CAD build for the part. Positions are in the model's coordinates, mm. Face numbers are marked on the shaded views. A direction names the side the tool comes from. Give positions to 0.01 mm unless a question says otherwise; leave off trailing zeros. Order: outer loops, then holes, each group sorted by start corner. A loop starts at its lowest first (then second) coordinate and runs counter-clockwise, first axis right, second up.
Item 1: Band-saw the part on B-B on y = 12. Give the cut face in (x, z), plus the area to 3 significant figures.
Item 2: Wall check: L1, parallel to X at y = -5.5, z = 15; L2, parallel to Y at x = 93.5, z = 23.5; L3, parallel to Y at x = -69, z = 2.25. Give the ranges that are in metal, low to high.
Item 3: Band-saw the part on A-A on z = 15. Give the cut face in (x, y).
Item 4: Which spindle directions (+Z, -Z, +X, -X, +Y, -Y) get a long thin tool onto all of the face, cutting with end or side? Do the marked faces 5, 6 and 7. Say none if no direction does.
Item 5: Band-saw the part on D-D on x = -52. Give the cut face in (y, z), plus the area to 3 significant figures.
Item 6: Flat gauge pins, fed straight in: P1, Ø5, axis at y = 53.5, z = 6.5, coming from the -X side; P2, Ø11, axis at y = 19, z = 7, coming from the +X side; P3, Ø1.5, axis at y = 42, z = 24.5, coming from the -X side; P4, Ø10, axis at x = 42, y = 9.5, coming from the +Z side. Where does each tip first touch, or does it go through?
Item 7: Band-saw the part on C-C on z = 5. Give the cut face in (x, y), plus the area to 3 significant figures.
Item 8: Two-plate mould, pull along Y, no slides. Class the marked faces 1, 2, 3 and 4: released by +Y, released by -Y, zero draft, split by the parting line, or undercut.
```python
from build123d import *

# Parameters (mm, degrees)
BOSS_EXTRUDE1_DEPTH = 30
SKETCH2_R           = 5
CUT_EXTRUDE1_DEPTH  = 90


with BuildPart() as part:
    # Sketch1 → Boss-Extrude1 (new body)
    with BuildSketch(Plane.XY):
        Polygon((-77.503184713, 15), (-77.503184713, -15), (102.496815287, -15), (102.496815287, 0), (72.496815287, 0), (72.496815287, 70.165605096), (102.496815287, 70.165605096), (102.496815287, 85.165605096), (52.496815287, 85.165605096), (-47.503184713, 15), align=None)
        with BuildLine():
            Line((52.496815287, 50.932984608), (52.496815287, 10))
            ThreePointArc((52.496815287, 10), (49.567883098, 2.928932188), (42.496815287, 0))
            Line((42.496815287, 0), (-15.840862486, 0))
            ThreePointArc((-15.840862486, 0), (-25.376570483, 6.988310608), (-21.58458061, 18.185945401))
            Line((-21.58458061, 18.185945401), (36.753097163, 59.11893001))
            ThreePointArc((36.753097163, 59.11893001), (47.109993083, 59.805334388), (52.496815287, 50.932984608))
        make_face(mode=Mode.SUBTRACT)
    extrude(amount=BOSS_EXTRUDE1_DEPTH)

    # Sketch2 → Cut-Extrude1 (cut, symmetric)
    with BuildSketch(Plane(origin=(0, 15, 0), x_dir=(1, 0, 0), z_dir=(0, 1, 0))):
        with Locations(Location((-62.503184713, -15, 0), (0, 0, 270))):
            Circle(SKETCH2_R)
        with Locations(Location((72.496815287, -15, 0), (0, 0, 270))):
            Circle(SKETCH2_R)
    extrude(amount=CUT_EXTRUDE1_DEPTH, both=True, mode=Mode.SUBTRACT)


solid = part.part
```
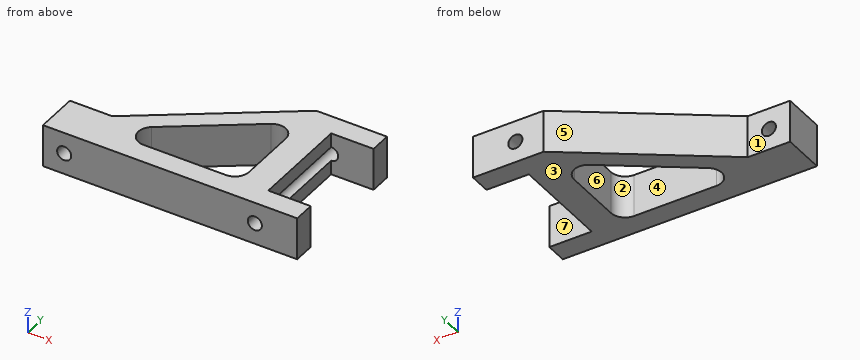
The answers:
1. outline: (-77.5, 0) - (-25.64, 0) - (-25.64, 30) - (-77.5, 30) - close; (52.5, 0) - (72.5, 0) - (72.5, 10) arc R5 cw to (72.5, 20) - (72.5, 30) - (52.5, 30) - close; hole circle Ø10 at (-62.5, 15)
1. area: 2,040 mm2
2. L1: x = -77.5 to -67.5, -57.5 to 67.5, 77.5 to 102.5
2. L2: y = -15 to 0, 70.17 to 85.17
2. L3: y = -15 to 15
3. outline: (-77.5, -15) - (-67.5, -15) - (-67.5, 15) - (-77.5, 15) - close; (-57.5, -15) - (67.5, -15) - (67.5, 85.17) - (52.5, 85.17) - (-47.5, 15) - (-57.5, 15) - close; (77.5, -15) - (102.5, -15) - (102.5, 0) - (77.5, 0) - close; (77.5, 70.17) - (102.5, 70.17) - (102.5, 85.17) - (77.5, 85.17) - close; hole (-21.58, 18.19) arc R10 ccw to (-15.84, 0) - (42.5, 0) arc R10 ccw to (52.5, 10) - (52.5, 50.93) arc R10 ccw to (36.75, 59.12) - close
4. face 5: +Z, -Z, -X, +Y
4. face 6: +Z, -Z
4. face 7: +Z, -Z, +X
5. outline: (-15, 0) - (15, 0) - (15, 30) - (-15, 30) - close
5. area: 900 mm2
6. P1: stops at x = 3.8
6. P2: stops at x = 72.5
6. P3: stops at x = -10.09
6. P4: passes through
7. outline: (-77.5, -15) - (102.5, -15) - (102.5, 0) - (72.5, 0) - (72.5, 70.17) - (102.5, 70.17) - (102.5, 85.17) - (52.5, 85.17) - (-47.5, 15) - (-77.5, 15) - close; hole (-21.58, 18.19) arc R10 ccw to (-15.84, 0) - (42.5, 0) arc R10 ccw to (52.5, 10) - (52.5, 50.93) arc R10 ccw to (36.75, 59.12) - close
7. area: 7,100 mm2
8. face 1: released by +Y
8. face 2: undercut
8. face 3: zero draft
8. face 4: undercut
